For this review, take the finished solid that the model builds, in its own axes (mm). A direction names the side the tool comes from. Coordinates: 2 decimals unless noted, no trailing zeros. Loops run counter-clockwise (first coordinate to the right, second up) from the corner with the lowest first, then second, coordinate; pieces in that order, holes last. Notation, with made-up numbers: (-20.75, 6) -> (19.25, 6) arc R23 ccw to (19.25, 23) -> close; hole circle Ø7 at (-21, 59.5). An arc over 180 degrees is marked (long way). Use a Markdown table: item, result.
from build123d import *

# Parameters (mm, degrees)
F0_R      = 44.5
F1_DEPTH  = 2
F2_R      = 44.5
F2_R_2    = 43.5
F3_DEPTH  = 15
F4_R      = 9
F5_DEPTH  = 25
F7_W      = 10
F7_H      = 1
F8_DEPTH  = 10
F10_W     = 10
F10_H     = 2
F11_DEPTH = 2
F12_SIZE  = 1.99999


# Not quite as in the source:
# - a fillet or chamfer is up to 0.001 mm smaller than in the source, because OpenCascade refuses the exact size


with BuildPart() as f1:
    # F0 (on Top) → F1 (new body)
    with BuildSketch(Plane.XY):
        Circle(F0_R)
    extrude(amount=F1_DEPTH)

    # F2 (on face) → F3 (join)
    with BuildSketch(Plane.XY.offset(2)):
        Circle(F2_R)
        Circle(F2_R_2, mode=Mode.SUBTRACT)
    extrude(amount=F3_DEPTH)

    # F4 (on face) → F5 (cut)
    with BuildSketch(Plane.XY.offset(2)):
        Circle(F4_R)
    extrude(amount=-F5_DEPTH, mode=Mode.SUBTRACT)

    # F7 (on face) → F8 (join)
    with BuildSketch(Plane.XY.offset(2)):
        with Locations((0, 28)):
            Rectangle(F7_W, F7_H)
        with Locations((0, -28)):
            Rectangle(F7_W, F7_H)
    extrude(amount=F8_DEPTH)

    # F10 (on face) → F11 (join)
    with BuildSketch(Plane.XZ.offset(-27.5)):
        with Locations((0, 11)):
            Rectangle(F10_W, F10_H)
    extrude(amount=F11_DEPTH)

    # F12 (size 2 in the source; OpenCascade refuses exactly that, so slightly less here)
    f12_edges = [f1.edges().sort_by_distance(p)[0] for p in [
        (0, 25.5, 12),
    ]]
    chamfer(f12_edges, length=F12_SIZE)


solid = f1.part
(1) Take a section at D-D on z = 15. Write out the cut boundary in (x, y).
Found:
| item | result |
|---|---|
| outline | circle Ø89 at (0, 0); hole circle Ø87 at (0, 0) |
(2) For faces 1 (the face through (0, 27, 10)), 2 (the face through (-32.798, 30.075, 8.381)), 3 (the face through (-5, 28, 8)), list the 3-axis set-ups (+Z, -Z, +X, -X, +Y, -Y) from which the entire face can be reached by the end or side of a thin tool; tool diameter is ignored.
Found:
| item | result |
|---|---|
| face 1 | none |
| face 2 | +Z, -Z |
| face 3 | +Z |
(3) For pin 1 Ø0.8 at (y, z) = (-28, 7.5) entering from +X; pin 2 Ø0.8 at (x, y) = (-1, 28) entering from +Z; pin 3 Ø0.9 at (y, z) = (27.5, 6.5) entering from -X; pin 4 Ø1.5 at (x, y) = (-12.5, 5.5) entering from -Z, all flat-tipped, find the tip position at first contact; note any pin that passes through.
Found:
| item | result |
|---|---|
| pin 1 | stops at x = 34.91 |
| pin 2 | stops at z = 12 |
| pin 3 | stops at x = -35.33 |
| pin 4 | stops at z = 0 |
(4) Take a section at C-C on y = 13.5. Write out the cut boundary in (x, z), plus the area to 3 significant figures.
Found:
| item | result |
|---|---|
| outline | (-42.4, 0) -> (42.4, 0) -> (42.4, 17) -> (41.35, 17) -> (41.35, 2) -> (-41.35, 2) -> (-41.35, 17) -> (-42.4, 17) -> close |
| area | 201 mm^2 |
(5) Take a section at B-B on y = 0. Write out the cut boundary in (x, z), plus the area to 3 significant figures.
Found:
| item | result |
|---|---|
| outline | (-44.5, 0) -> (-9, 0) -> (-9, 2) -> (-43.5, 2) -> (-43.5, 17) -> (-44.5, 17) -> close; (9, 0) -> (44.5, 0) -> (44.5, 17) -> (43.5, 17) -> (43.5, 2) -> (9, 2) -> close |
| area | 172 mm^2 |
(6) For line 1 along Y through (x, z) = (0, 8.5); line 2 along Y through (x, z) = (0, 1.55); line 3 along Y through (x, z) = (0, 12.25), list the stretches that pass through material, from the lowest coordinate up.
Found:
| item | result |
|---|---|
| line 1 | y = -44.5 to -43.5, -28.5 to -27.5, 27.5 to 28.5, 43.5 to 44.5 |
| line 2 | y = -44.5 to -9, 9 to 44.5 |
| line 3 | y = -44.5 to -43.5, 43.5 to 44.5 |
(7) Mouldability with a two-part tool opening along Z and no side actions: class faces 4 (the face through (0, 27.5, 6)), 5 (the face through (-0.6, -9.3, 0)), 6 (the face through (-5.66, 43.13, 9.4)), 7 (the face through (10, -43, 17)) as pulls with the +Z half, pulls with the -Z half, needs draft (parallel to the pull), parting line crosses it, or undercut.
Found:
| item | result |
|---|---|
| face 4 | undercut |
| face 5 | pulls with the -Z half |
| face 6 | needs draft |
| face 7 | pulls with the +Z half |
